from build123d import *

# Parameters (mm, degrees)
F0_W     = 55
F0_H     = 40
F0_R     = 2
F1_DEPTH = 5
F2_W     = 7
F2_H     = 40
F3_DEPTH = 55
F4_R     = 1
F5_DEPTH = 15
F6_R     = 5
F7_W     = 5
F7_H     = 5
F8_DEPTH = 40
F9_SIZE  = 4.99999


# Not quite as in the source:
# - a fillet or chamfer is up to 0.001 mm smaller than in the source, because OpenCascade refuses the exact size


with BuildPart() as f1:
    # F0 (on Top) → F1 (new body)
    with BuildSketch(Plane.XY):
        Rectangle(F0_W, F0_H)
        with Locations((-12.5, -10)):
            Circle(F0_R, mode=Mode.SUBTRACT)
        with Locations((12.5, -10)):
            Circle(F0_R, mode=Mode.SUBTRACT)
        with Locations((-12.5, 10)):
            Circle(F0_R, mode=Mode.SUBTRACT)
        with Locations((12.5, 10)):
            Circle(F0_R, mode=Mode.SUBTRACT)
    extrude(amount=F1_DEPTH)

    # F2 (on face) → F3 (join)
    with BuildSketch(Plane.XY.offset(5)):
        with Locations((-24, 0)):
            Rectangle(F2_W, F2_H)
        with Locations((24, 0)):
            Rectangle(F2_W, F2_H)
    extrude(amount=F3_DEPTH)

    # F4 (on face) → F5 (cut)
    with BuildSketch(Plane.XY.offset(60)):
        with Locations((-24, 9.358282201)):
            Circle(F4_R)
        with Locations((24, 9.358282201)):
            Circle(F4_R)
        with Locations((24, -9.358282201)):
            Circle(F4_R)
        with Locations((-24, -9.358282201)):
            Circle(F4_R)
    extrude(amount=-F5_DEPTH, mode=Mode.SUBTRACT)

    # F6
    f6_edges = [f1.edges().sort_by_distance(p)[0] for p in [
        (-27.5, 20, 30),
        (-27.5, -20, 30),
        (27.5, -20, 30),
        (27.5, 20, 30),
    ]]
    fillet(f6_edges, radius=F6_R)

    # F7 (on face) → F8 (join)
    with BuildSketch(Plane(origin=(0, 20, 0), x_dir=(-1, 0, 0), z_dir=(0, 1, 0))):
        with Locations((-18, 7.5)):
            Rectangle(F7_W, F7_H)
        with Locations((18, 7.5)):
            Rectangle(F7_W, F7_H)
    extrude(amount=-F8_DEPTH)

    # F9 (size 5 in the source; OpenCascade refuses exactly that, so slightly less here)
    f9_edges = [f1.edges().sort_by_distance(p)[0] for p in [
        (15.5, 0, 10),
        (-15.5, 0, 10),
    ]]
    chamfer(f9_edges, length=F9_SIZE)


solid = f1.part
For this review, take the finished solid that the model builds, in its own axes (mm). A direction names the side the tool comes from. Round coordinates to 2 decimals unless told otherwise and drop trailing zeros. Write each loop counter-clockwise with the first axis right and the second up, starting at its lowest first coordinate (ties: lowest second). Pieces come first, ordered by that corner, then holes. Notation, with made-up numbers: (-40, 52.5) - (18, 52.5) arc R31 cw to (18, 91.5) - close; hole circle Ø2 at (-11.5, 23). An arc over 180 degrees is marked (long way). Use a Markdown table: item, result.
Q1. Clearance check with flat-ended pins moving along their axes: pin 1 (6 mm diameter, centred on x = 6, y = 5.5, fed in from +Z); pin 2 (1.6 mm diameter, centred on x = -24, y = 9.36, fed in from +Z). State where each tip first meets the part, or that it passes through.
Derived:
| item | result |
|---|---|
| pin 1 | stops at z = 5 |
| pin 2 | stops at z = 45 |
Q2. The part is to be moulded in two halves that separate along X. For faces 4 (the cylindrical face through (11.026, 11.352, 2.465)), 5 (the cylindrical face through (-26.07, 18.5, 29.58)), 6 (the cylindrical face through (26, -18.57, 30.42)), say which applies: pulls with the +X half, pulls with the -X half, needs draft (parallel to the pull), parting line crosses it, or undercut.
Derived:
| item | result |
|---|---|
| face 4 | undercut |
| face 5 | pulls with the -X half |
| face 6 | pulls with the +X half |
Q3. We need section A-A (x = 12.5). Give the boundary of the cut face in (y, z).
Derived:
| item | result |
|---|---|
| outline | (-20, 0) - (-12, 0) - (-12, 5) - (-20, 5) - close; (-8, 0) - (8, 0) - (8, 5) - (-8, 5) - close; (12, 0) - (20, 0) - (20, 5) - (12, 5) - close |
Q4. Wall thickness on line 1 along Y through (x, z) = (12.5, 2.15); line 2 along X through (y, z) = (10, 28.5); line 3 along X through (y, z) = (9.5, 47): over which ranges is each line inside the solid? List them lowest first.
Derived:
| item | result |
|---|---|
| line 1 | y = -20 to -12, -8 to 8, 12 to 20 |
| line 2 | x = -27.5 to -20.5, 20.5 to 27.5 |
| line 3 | x = -27.5 to -24.99, -23.01 to -20.5, 20.5 to 23.01, 24.99 to 27.5 |
Q5. We need section D-D (z = 47.5). Give the boundary of the cut face in (x, y).
Derived:
| item | result |
|---|---|
| outline | (-27.5, -15) arc R5 ccw to (-22.5, -20) - (-20.5, -20) - (-20.5, 20) - (-22.5, 20) arc R5 ccw to (-27.5, 15) - close; (20.5, -20) - (22.5, -20) arc R5 ccw to (27.5, -15) - (27.5, 15) arc R5 ccw to (22.5, 20) - (20.5, 20) - close; hole circle Ø2 at (-24, -9.36); hole circle Ø2 at (-24, 9.36); hole circle Ø2 at (24, -9.36); hole circle Ø2 at (24, 9.36) |
Q6. We need section B-B (z = 24.5). Give the boundary of the cut face in (x, y).
Derived:
| item | result |
|---|---|
| outline | (-27.5, -15) arc R5 ccw to (-22.5, -20) - (-20.5, -20) - (-20.5, 20) - (-22.5, 20) arc R5 ccw to (-27.5, 15) - close; (20.5, -20) - (22.5, -20) arc R5 ccw to (27.5, -15) - (27.5, 15) arc R5 ccw to (22.5, 20) - (20.5, 20) - close |
Q7. Machinability: for faces 1 (the flat face through (-18, 0.3, 7.5)), 2 (the flat face through (-24, 9, 45)), 3 (the cylindrical face through (11.026, -8.648, 2.465)), which of the approach directions +Z, -Z, +X, -X, +Y, -Y give a long, thin tool a straight path to every point of the face, cutting with its end or side? Answer none if there is none.
Derived:
| item | result |
|---|---|
| face 1 | +Z, +Y, -Y |
| face 2 | +Z |
| face 3 | +Z, -Z |
